```python
from build123d import *

# Parameters (mm, degrees)
F0_W     = 254
F0_H     = 203.2
F0_R     = 7.14375
F1_DEPTH = 12.7
F2_W     = 254
F2_H     = 203.2
F2_R     = 7.14375
F3_DEPTH = 12.7
F4_W     = 254
F4_H     = 12.7
F5_DEPTH = 50.8
F6_SIZE  = 38.1
F7_W     = 254
F7_H     = 12.7
F8_DEPTH = 50.8
F9_SIZE  = 38.1
F10_SIZE = 6.35


with BuildPart() as f1:
    # F0 (on Top) → F1 (new body)
    with BuildSketch(Plane.XY):
        with Locations((-76.2, 0)):
            Rectangle(F0_W, F0_H)
        with Locations((-184.15, -82.55)):
            Circle(F0_R, mode=Mode.SUBTRACT)
        with Locations((-95.25, -82.55)):
            Circle(F0_R, mode=Mode.SUBTRACT)
        with Locations((-184.15, 82.55)):
            Circle(F0_R, mode=Mode.SUBTRACT)
        with Locations((-95.25, 82.55)):
            Circle(F0_R, mode=Mode.SUBTRACT)
    extrude(amount=F1_DEPTH)

    # F2 (on face) → F3 (join)
    with BuildSketch(Plane(origin=(0, 0, 0), x_dir=(1, 0, 0), z_dir=(0, 0, -1))):
        with Locations((76.2, 0)):
            Rectangle(F2_W, F2_H)
        with Locations((95.25, -82.55)):
            Circle(F2_R, mode=Mode.SUBTRACT)
        with Locations((184.15, -82.55)):
            Circle(F2_R, mode=Mode.SUBTRACT)
        with Locations((95.25, 82.55)):
            Circle(F2_R, mode=Mode.SUBTRACT)
        with Locations((184.15, 82.55)):
            Circle(F2_R, mode=Mode.SUBTRACT)
    extrude(amount=F3_DEPTH)

    # F4 (on face) → F5 (join)
    with BuildSketch(Plane.XY.offset(12.7)):
        with Locations((-76.2, 0)):
            Rectangle(F4_W, F4_H)
    extrude(amount=F5_DEPTH)

    # F6
    f6_edges = [f1.edges().sort_by_distance(p)[0] for p in [
        (-203.2, 0, 63.5),
        (50.8, 0, 63.5),
    ]]
    chamfer(f6_edges, length=F6_SIZE)

    # F7 (on face) → F8 (join)
    with BuildSketch(Plane(origin=(0, 0, -12.7), x_dir=(1, 0, 0), z_dir=(0, 0, -1))):
        with Locations((76.2, 0)):
            Rectangle(F7_W, F7_H)
    extrude(amount=F8_DEPTH)

    # F9
    f9_edges = [f1.edges().sort_by_distance(p)[0] for p in [
        (203.2, 0, -63.5),
        (-50.8, 0, -63.5),
    ]]
    chamfer(f9_edges, length=F9_SIZE)

    # F10
    f10_edges = [f1.edges().sort_by_distance(p)[0] for p in [
        (50.8, 0, 0),
        (-76.2, -6.35, 12.7),
        (-76.2, 6.35, 12.7),
        (-50.8, 0, 0),
        (76.2, 6.35, -12.7),
        (76.2, -6.35, -12.7),
    ]]
    chamfer(f10_edges, length=F10_SIZE)


solid = f1.part
```
Work out the finished part from the listing and answer in its coordinate system (mm). A direction names the side the tool comes from. Coordinates: 2 decimals unless noted, no trailing zeros. Order: outer loops, then holes, each group sorted by start corner. A loop starts at its lowest first (then second) coordinate and runs counter-clockwise, first axis right, second up. Notation, with made-up numbers: (-37.75, 45) - (12.25, 45) arc R24 cw to (12.25, 62) - close; hole circle Ø10 at (58, 80.25). An arc over 180 degrees is marked (long way). Answer as a JSON object with one key per item and string values.
1. A tool of negligible diameter and unlimited length cuts with its end or side. For faces 4 (the face through (-78, 58, 12.7)), 5 (the face through (-50.8, 1, -12)), 6 (the face through (129, -1, 0)), from which of +Z, -Z, +X, -X, +Y, -Y can it reach the whole face along a straight path? Write none if from no direction.
Output values:
{"face 4": "+Z, +X, -X, +Y", "face 5": "-Z, -X, +Y, -Y", "face 6": "+Z, +X, +Y, -Y"}
2. Each of these flat-tipped pins is pushed along its axis until it touches: P1, Ø5, axis at y = 5.5, z = 48.5, coming from the +X side; P2, Ø6, axis at x = -18, y = 69.5, coming from the -Z side; P3, Ø13.5, axis at x = 113.5, z = -44, coming from the -Y side. Where does it stop, or does it pass through?
Output values:
{"P1": "stops at x = 30.2", "P2": "stops at z = -12.7", "P3": "stops at y = -6.35"}
3. Find section A-A on y = -82.55. Determine the outline of the cut face in (x, z), plus the area to 3 significant figures.
Output values:
{"outline": "(-203.2, 0) - (-191.29, 0) - (-191.29, 12.7) - (-203.2, 12.7) - close; (-177.01, 0) - (-102.39, 0) - (-102.39, 12.7) - (-177.01, 12.7) - close; (-88.11, 0) - (-57.15, 0) - (-50.8, -6.35) - (-50.8, -12.7) - (88.11, -12.7) - (88.11, 0) - (57.15, 0) - (50.8, 6.35) - (50.8, 12.7) - (-88.11, 12.7) - close; (102.39, -12.7) - (177.01, -12.7) - (177.01, 0) - (102.39, 0) - close; (191.29, -12.7) - (203.2, -12.7) - (203.2, 0) - (191.29, 0) - close", "area": "5,770 mm²"}
4. Find section C-C on x = -31. Determine the outline of the cut face in (y, z).
Output values:
{"outline": "(-101.6, -12.7) - (-12.7, -12.7) - (-6.35, -19.05) - (-6.35, -45.2) - (6.35, -45.2) - (6.35, -19.05) - (12.7, -12.7) - (101.6, -12.7) - (101.6, 12.7) - (12.7, 12.7) - (6.35, 19.05) - (6.35, 63.5) - (-6.35, 63.5) - (-6.35, 19.05) - (-12.7, 12.7) - (-101.6, 12.7) - close"}
5. Consider line 1 (X direction, y = -82, z = 9); line 2 (Y direction, x = -95.25, z = 8.25); line 3 (X direction, y = -82, z = -6). Determine where each line is inside the solid, lowest interval first.
Output values:
{"line 1": "x = -203.2 to -191.27, -177.03 to -102.37, -88.13 to 50.8", "line 2": "y = -101.6 to -89.69, -75.41 to 75.41, 89.69 to 101.6", "line 3": "x = -51.15 to 88.13, 102.37 to 177.03, 191.27 to 203.2"}
6. Find section B-B on x = 184.15. Determine the outline of the cut face in (y, z), plus the area to 3 significant figures.
Output values:
{"outline": "(-101.6, -12.7) - (-89.69, -12.7) - (-89.69, 0) - (-101.6, 0) - close; (-75.41, -12.7) - (-12.7, -12.7) - (-6.35, -19.05) - (-6.35, -44.45) - (6.35, -44.45) - (6.35, -19.05) - (12.7, -12.7) - (75.41, -12.7) - (75.41, 0) - (-75.41, 0) - close; (89.69, -12.7) - (101.6, -12.7) - (101.6, 0) - (89.69, 0) - close", "area": "2,660 mm²"}
7. Find section D-D on y = 27.5. Determine the outline of the cut face in (x, z).
Output values:
{"outline": "(-203.2, 0) - (-57.15, 0) - (-50.8, -6.35) - (-50.8, -12.7) - (203.2, -12.7) - (203.2, 0) - (57.15, 0) - (50.8, 6.35) - (50.8, 12.7) - (-203.2, 12.7) - close"}
8. The mould has two halves that part along Y. Classify faces 1 (the face through (31.5, -0.1, 44.7)), 2 (the face through (88.113, 82.236, -6.261)), 3 (the face through (-78, 6.35, 41)): +Y half, -Y half, draft (parallel to the pull), parting line (faces both ways), or undercut.
Output values:
{"face 1": "draft", "face 2": "undercut", "face 3": "+Y half"}
